```python
from build123d import *

# Parameters (mm, degrees)
CHANFREIN1_SIZE              = 0.3
ESQUISSE2_R                  = 4
ENL_V_MAT_EXTRU_1_DEPTH      = 2
R_P_TITION_CIRCULAIRE1_COUNT = 5


with BuildPart() as part:
    # Esquisse1 → Révolution1 (revolve)
    with BuildSketch(Plane.XY):
        with BuildLine():
            Line((-0.38, 0), (-2.5, 0))
            Line((-2.5, 0), (-2.5, 1))
            Line((-2.5, 1), (-4, 1))
            Line((-4, 1), (-4, 3))
            Line((-4, 3), (-2.985871259, 3))
            ThreePointArc((-2.985871259, 3), (-1.71951066, 3.492907341), (-0.38, 3.721682356))
            Line((-0.38, 3.721682356), (-0.38, 3))
            Line((-0.38, 3), (-0.38, 0))
        make_face()
    revolve(axis=Axis((0, 0, 0), (0, 1, 0)))

    # Chanfrein1
    chanfrein1_edges = [part.edges().sort_by_distance(p)[0] for p in [
        (2.5, 0, 0),
        (4, 3, 0),
        (4, 1, 0),
    ]]
    chamfer(chanfrein1_edges, length=CHANFREIN1_SIZE)

    # Esquisse2 → Enlèv. mat.-Extru.1 (cut)
    with BuildSketch(Plane(origin=(0, 3, 0), x_dir=(1, 0, 0), z_dir=(0, 1, 0))):
        with Locations((0, 7)):
            Circle(ESQUISSE2_R)
    enl_v_mat_extru_1 = extrude(amount=-ENL_V_MAT_EXTRU_1_DEPTH, mode=Mode.SUBTRACT)

    # Répétition circulaire1: Enlèv. mat.-Extru.1 ×5 about axis
    r_p_tition_circulaire1_axis = Axis((0, 0, 0), (0, 1, 0))
    for i in range(1, R_P_TITION_CIRCULAIRE1_COUNT):
        add(enl_v_mat_extru_1.rotate(r_p_tition_circulaire1_axis, i * 360 / R_P_TITION_CIRCULAIRE1_COUNT), mode=Mode.SUBTRACT)


solid = part.part
```
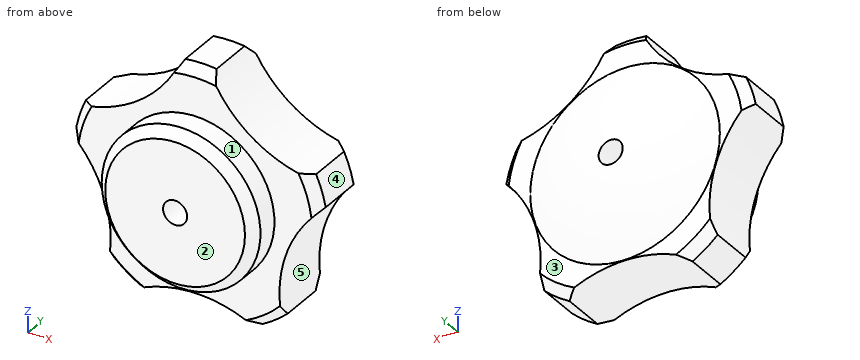
The listing builds one solid part. Answer for the finished solid, in the listing's coordinates (mm). Face numbers are marked on the shaded views. A direction names the side the tool comes from. Coordinates: 2 decimals unless noted, no trailing zeros. Write each loop counter-clockwise with the first axis right and the second up, starting at its lowest first coordinate (ties: lowest second). Pieces come first, ordered by that corner, then holes. Notation, with made-up numbers: M 69.5,37 L 86.5,37 A34 ccw 86.5,68 Z; hole C -11.5,42 d8. An arc over 180 degrees is marked long. Use a Markdown table: item, result. Add a question column.
1. Given P1, Ø1, axis at x = 1, z = 2, coming from the +Y side; P2, Ø1.5, axis at y = 2.5, z = -1, coming from the +X side; P3, Ø1.5, axis at y = 3.5, z = -1, coming from the -X side, each flat-ended and moving along its own axis, determine where each tip first touches the part or whether it passes through.
2. Section A-A (y = 1.95) is taken. Give the vertices of the cut face in (x, z), plus the area to 3 significant figures.
3. Which of the six approach directions +Z, -Z, +X, -X, +Y, -Y give full straight-line access (tool end or side, diameter ignored) to the marked faces 1 and 2?
4. Section C-C (z = 3.5) is taken. Give the vertices of the cut face in (x, y), plus the area to 3 significant figures.
5. Straight lines are drawn through the part: line 1 along Z through (x, y) = (0, 2.1); line 2 along Z through (x, y) = (0, 0.95); line 3 along Y through (x, z) = (-3, 0.75). For each, find the intervals that lie inside material, in ascending order. Write a range as [from, to].
6. For a pull along Z with two mould halves and no side action, classify the marked faces 3, 4 and 5 as +Z half, -Z half, draft (parallel to the pull), parting line (faces both ways), or undercut.
7. Section B-B (y = 1.1) is taken. Give the vertices of the cut face in (x, z).
Data:
| question | item | result |
|---|---|---|
| 1 | P1 | stops at y = 3.49 |
| 1 | P2 | stops at x = 3.14 |
| 1 | P3 | stops at x = -3.05 |
| 2 | outline | M -3.93,0.76 A4 cw -2.73,-2.92 A4 ccw -1.94,-3.5 A4 cw 1.94,-3.5 A4 ccw 2.73,-2.92 A4 cw 3.93,0.76 A4 ccw 3.62,1.69 A4 cw 0.49,3.97 A4 ccw -0.49,3.97 A4 cw -3.62,1.69 A4 ccw Z; hole C 0,0 d0.76 |
| 2 | area | 36.7 mm2 |
| 3 | face 1 | -Y |
| 3 | face 2 | +Z, -Z, +X, -X, -Y |
| 4 | outline | M -0.75,1 L 0.75,1 L 0.75,3 L -0.75,3 Z |
| 4 | area | 3.00 mm2 |
| 5 | line 1 | z = [-3, -0.38], [0.38, 4] |
| 5 | line 2 | z = [-2.5, -0.38], [0.38, 2.5] |
| 5 | line 3 | y = [1, 3] |
| 6 | face 3 | draft |
| 6 | face 4 | +Z half |
| 6 | face 5 | undercut |
| 7 | outline | M -3.75,0.59 A4 cw -2.69,-2.68 A3.8 ccw -1.72,-3.39 A4 cw 1.72,-3.39 A3.8 ccw 2.69,-2.68 A4 cw 3.75,0.59 A3.8 ccw 3.38,1.73 A4 cw 0.6,3.75 A3.8 ccw -0.6,3.75 A4 cw -3.38,1.73 A3.8 ccw Z; hole C 0,0 d0.76 |
